Read the model definition and answer for the solid it produces. Units are mm, in the model's axes. A direction names the side the tool comes from. Coordinates: 2 decimals unless noted, no trailing zeros. Write each loop counter-clockwise with the first axis right and the second up, starting at its lowest first coordinate (ties: lowest second). Pieces come first, ordered by that corner, then holes. Notation, with made-up numbers: (5, -22.75) -> (45, -22.75) arc R27 cw to (45, 15.25) -> close; hole circle Ø7 at (-20.75, 45). An arc over 180 degrees is marked (long way). Return JSON: item names as keys, results as strings.
from build123d import *

# Parameters (mm, degrees)
F1_DEPTH = 50.8
F2_W     = 64.513084
F2_H     = 66.808922
F3_DEPTH = 5.08


with BuildPart() as f1:
    # F0 (on Front) → F1 (new body)
    with BuildSketch(Plane.XZ):
        with BuildLine():
            ThreePointArc((-39.832812, 33.289671), (-43.655486, 40.201062), (-51.541593, 40.636353))
            Line((-51.541593, 40.636353), (-51.541593, -26.402151))
            Line((-51.541593, -26.402151), (-39.832812, -26.402151))
            Line((-39.832812, -26.402151), (-39.832812, -17.163772))
            Line((-39.832812, -17.163772), (-39.832812, 33.289671))
        make_face()
        with BuildLine():
            Line((-39.832812, -17.163772), (-39.832812, -26.402151))
            Line((-39.832812, -26.402151), (10.788094, -26.402151))
            ThreePointArc((10.788094, -26.402151), (15.407284, -21.782962), (10.788094, -17.163772))
            Line((10.788094, -17.163772), (-39.832812, -17.163772))
        make_face()
    extrude(amount=F1_DEPTH)

    # F2 (on Front) → F3 (join)
    with BuildSketch(Plane.XZ):
        with Locations((-19.055465, 7.00231)):
            Rectangle(F2_W, F2_H)
    extrude(amount=F3_DEPTH)


solid = f1.part
1. A tool of negligible diameter and unlimited length cuts with its end or side. For faces 1 (the face through (-9, -5.08, 12)), 2 (the face through (-41, -50.8, -5)), 3 (the face through (-43.56, -25.04, 40.14)), 4 (the face through (-16, -3, 40.407)), 5 (the face through (15.406, -25.044, -21.885)), from which of +Z, -Z, +X, -X, +Y, -Y can it reach the whole face along a straight path? Write none if from no direction.
Taken from the geometry:
{"face 1": "+Z, +X, -Y", "face 2": "+Z, -Z, +X, -X, -Y", "face 3": "+Z, -Y", "face 4": "+Z, +X, +Y, -Y", "face 5": "+X, -Y"}
2. The part is cut by section A-A (y = -32.5). Determine the outline of the cut face in (x, z), then the cut area to 3 significant figures.
Taken from the geometry:
{"outline": "(-51.54, -26.4) -> (10.79, -26.4) arc R4.62 ccw to (10.79, -17.16) -> (-39.83, -17.16) -> (-39.83, 33.29) arc R8.16 ccw to (-51.54, 40.64) -> close", "area": "1,280 mm2"}
3. Flat-ended cylindrical pins translate along their axes: pin 1 Ø13.5 at (y, z) = (-18.5, 5) entering from +X; pin 2 Ø2.5 at (y, z) = (-2, 8) entering from +X; pin 3 Ø4 at (x, y) = (-23.5, -2.5) entering from +Z; pin 4 Ø1.5 at (x, z) = (-36, -3.5) entering from +Y. Find the tip coordinate at first contact, or state that the pin passes through.
Taken from the geometry:
{"pin 1": "stops at x = -39.83", "pin 2": "stops at x = 13.2", "pin 3": "stops at z = 40.41", "pin 4": "stops at y = 0"}
4. Consider L1, parallel to Y at x = -1.5, z = 30; L2, parallel to X at y = -9.5, z = 14.5; L3, parallel to Z at x = -34.5, y = -9.5. Determine where each line is inside the solid, lowest interval first.
Taken from the geometry:
{"L1": "y = -5.08 to 0", "L2": "x = -51.54 to -39.83", "L3": "z = -26.4 to -17.16"}
5. The part is cut by section B-B (x = -6.5). Determine the outline of the cut face in (y, z).
Taken from the geometry:
{"outline": "(-50.8, -26.4) -> (0, -26.4) -> (0, 40.41) -> (-5.08, 40.41) -> (-5.08, -17.16) -> (-50.8, -17.16) -> close"}
